The listing builds one solid part. Answer for the finished solid, in the listing's coordinates (mm). Round coordinates to 2 decimals unless told otherwise and drop trailing zeros. Order: outer loops, then holes, each group sorted by start corner. A loop starts at its lowest first (then second) coordinate and runs counter-clockwise, first axis right, second up. Notation, with made-up numbers: M 38.25,-35 L 95.25,-35 A24 ccw 95.25,-11 Z; hole C -12,66.5 d11. An arc over 180 degrees is marked long. Put each result on its own line as item: value. Start each with the question number.
1. The part is cut by section C-C (z = -1.5). Give the vertices of the cut face in (x, y).
2. Consider line 1 (Y direction, x = 20, z = -4); line 2 (X direction, y = 5.5, z = -3.5); line 3 (X direction, y = 9, z = -0.25). Determine where each line is inside the solid, lowest interval first.
3. Each of these flat-tipped pins is pushed along its axis until it touches: pin 1 Ø1.5 at (y, z) = (11, -1.5) entering from -X; pin 2 Ø1 at (y, z) = (9, -2.5) entering from -X. Where does it stop, or does it pass through?
4. The mould has two halves that part along Y. Classify faces 1 (the face through (115, 0, -3)), 2 (the face through (214.977, 6.542, -3.131)), 3 (the face through (230.86, 7.6, -3.13)): +Y half, -Y half, draft (parallel to the pull), parting line (faces both ways), or undercut.
5. The part is cut by section A-A (x = 20). Give the vertices of the cut face in (y, z), then the cut area to 3 significant figures.
6. The part is cut by section B-B (y = 7.5). Give the vertices of the cut face in (x, z).
from build123d import *

# Parameters (mm, degrees)
SKETCH1_W           = 232.6676516
SKETCH1_H           = 15
BOSS_EXTRUDE1_DEPTH = 6.35
CUT_EXTRUDE1_DEPTH  = 234.237129551
SKETCH3_R           = 2.5
CUT_EXTRUDE2_DEPTH  = 234.237129551


with BuildPart() as part:
    # Sketch1 → Boss-Extrude1 (new body)
    with BuildSketch(Plane.XY):
        with Locations((116.3338258, 7.5)):
            Rectangle(SKETCH1_W, SKETCH1_H)
    extrude(amount=-BOSS_EXTRUDE1_DEPTH)

    # Sketch2 → Cut-Extrude1 (cut, through all)
    with BuildSketch(Plane(origin=(0, 15, 0), x_dir=(1, 0, 0), z_dir=(0, 1, 0))):
        Polygon((0, 0), (0, 6.35), (3.666174209, 6.35), align=None)
        Polygon((232.6676516, 0), (229.001477391, 6.35), (232.6676516, 6.35), align=None)
    extrude(amount=-CUT_EXTRUDE1_DEPTH, mode=Mode.SUBTRACT)

    # Sketch3 → Cut-Extrude2 (cut, through all)
    with BuildSketch(Plane.XY):
        with Locations((20, 7.5)):
            Circle(SKETCH3_R)
        with Locations((212.6676516, 7.5)):
            Circle(SKETCH3_R)
    extrude(amount=-CUT_EXTRUDE2_DEPTH, mode=Mode.SUBTRACT)


solid = part.part
Resolved:
1. outline: M 0.87,0 L 231.8,0 L 231.8,15 L 0.87,15 Z; hole C 20,7.5 d5; hole C 212.67,7.5 d5
2. line 1: 0 to 5, 10 to 15
2. line 2: 2.02 to 18.5, 21.5 to 211.17, 214.17 to 230.65
2. line 3: 0.14 to 18, 22 to 210.67, 214.67 to 232.52
3. pin 1: x = 0.43
3. pin 2: x = 1.15
4. face 1: -Y half
4. face 2: undercut
4. face 3: draft
5. outline: M 0,-6.35 L 5,-6.35 L 5,0 L 0,0 Z; M 10,-6.35 L 15,-6.35 L 15,0 L 10,0 Z
5. area: 63.5 mm2
6. outline: M 0,0 L 3.67,-6.35 L 17.5,-6.35 L 17.5,0 Z; M 22.5,-6.35 L 210.17,-6.35 L 210.17,0 L 22.5,0 Z; M 215.17,-6.35 L 229,-6.35 L 232.67,0 L 215.17,0 Z
